Verification items for the finished model (mm, model axes). Face numbers are marked on the shaded views. A direction names the side the tool comes from. Give positions to 0.01 mm unless a question says otherwise; leave off trailing zeros. Order: outer loops, then holes, each group sorted by start corner. A loop starts at its lowest first (then second) coordinate and runs counter-clockwise, first axis right, second up. Notation, with made-up numbers: (2.25, 29) - (15.25, 29) arc R28 cw to (15.25, 47) - close; hole circle Ø11 at (12.5, -18). An arc over 180 degrees is marked (long way). Answer as a JSON object with one key per item and string values.
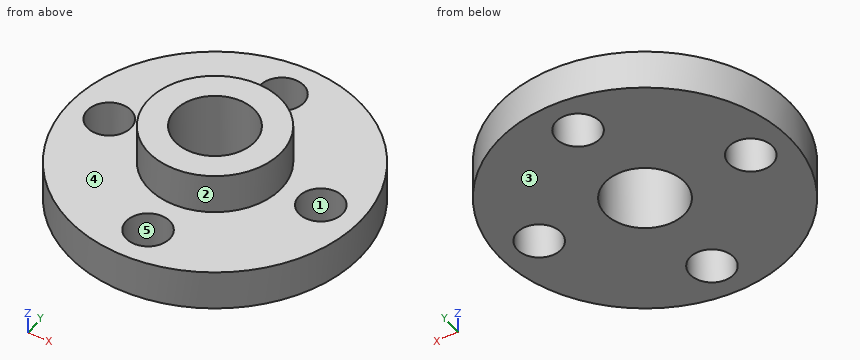
Autodesk Inventor part; units mm, degrees
ref_plane "YZ Plane" through (0, 0, 0) normal (1, 0, 0) x (0, 1, 0)
ref_plane "XZ Plane" through (0, 0, 0) normal (0, 1, 0) x (-1, 0, 0)
ref_plane "XY Plane" through (0, 0, 0) normal (0, 0, 1) x (1, 0, 0)
sketch "Sketch1" plane through (0, 0, 0) normal (0, 0, 1) x (1, 0, 0)
  circle A0 centre (0, 0) radius 11
  circle A1 centre (0, 8) radius 1.65
  line L0 (-3.4226, 0) -> (4.8397, 0) construction
  line L1 (0, 0) -> (0, 2.4255) construction
  circle A2 centre (8, 0) radius 1.65
  circle A3 centre (0, -8) radius 1.65
  circle A4 centre (-8, 0) radius 1.65
  dimension "d0" = 22
  dimension "d1" = 8
  dimension "d2" = 3.3
  dimension "d3" = 8
  dimension "d4" = 3.3
extrude "Extrusion1" add sketch "Sketch1" along normal blind 3
sketch "Sketch2" plane through (0, 0, 3) normal (0, 0, 1) x (1, 0, 0)
  circle A0 centre (0, 0) radius 5
  dimension "d7" = 10
extrude "Extrusion2" add sketch "Sketch2" along normal blind 3
sketch "Sketch3" plane through (0, 0, 6) normal (0, 0, 1) x (1, 0, 0)
  circle A0 centre (0, 0) radius 3
  dimension "d10" = 6
extrude "Extrusion3" cut sketch "Sketch3" against normal through all
equation "\"d4\" = d2"
properties part number "Acople" material "ABS Plastic"
(1) Section check D-D (y = 9). Record the cut outline in (x, z), then the cut area to 3 significant figures.
Computed values:
{"outline": "(-6.32, 0) - (-1.31, 0) - (-1.31, 3) - (-6.32, 3) - close; (1.31, 0) - (6.32, 0) - (6.32, 3) - (1.31, 3) - close", "area": "30.1 mm²"}
(2) Section check B-B (z = 0.65). Record the cut outline in (x, y), then the cut area to 3 significant figures.
Computed values:
{"outline": "circle Ø22 at (0, 0); hole circle Ø3.3 at (-8, 0); hole circle Ø6 at (0, 0); hole circle Ø3.3 at (0, -8); hole circle Ø3.3 at (0, 8); hole circle Ø3.3 at (8, 0)", "area": "318 mm²"}
(3) Gauge pin test, flat ends, axial feed: pin 1 Ø4.5 at (x, y) = (0, 8) entering from -Z; pin 2 Ø2 at (y, z) = (8, 3) entering from -X; pin 3 Ø4.5 at (x, y) = (0, -8) entering from +Z; pin 4 Ø1.5 at (y, z) = (7, 3) entering from -X. Record the tip position at first contact, or that the pin passes through.
Computed values:
{"pin 1": "stops at z = 0", "pin 2": "stops at x = -8.49", "pin 3": "stops at z = 3", "pin 4": "stops at x = -9.05"}
(4) Section check C-C (x = 8.25). Record the cut outline in (y, z).
Computed values:
{"outline": "(-7.28, 0) - (-1.63, 0) - (-1.63, 3) - (-7.28, 3) - close; (1.63, 0) - (7.28, 0) - (7.28, 3) - (1.63, 3) - close"}
(5) Section check A-A (x = 0). Record the cut outline in (y, z), then the cut area to 3 significant figures.
Computed values:
{"outline": "(-11, 0) - (-9.65, 0) - (-9.65, 3) - (-11, 3) - close; (-6.35, 0) - (-3, 0) - (-3, 6) - (-5, 6) - (-5, 3) - (-6.35, 3) - close; (3, 0) - (6.35, 0) - (6.35, 3) - (5, 3) - (5, 6) - (3, 6) - close; (9.65, 0) - (11, 0) - (11, 3) - (9.65, 3) - close", "area": "40.2 mm²"}
(6) Release check for a two-part mould opening along X. For the marked faces 1, 2 and 3 record: pulls with the +X half, pulls with the -X half, needs draft (parallel to the pull), parting line crosses it, or undercut.
Computed values:
{"face 1": "undercut", "face 2": "parting line crosses it", "face 3": "needs draft"}
(7) Material ranges on line 1 along Y through (x, z) = (0, 1.3); line 2 along X through (y, z) = (-1.25, 1.2); line 3 along X through (y, z) = (0.25, 2.4), recorded low to high. Write a range as [from, to].
Computed values:
{"line 1": "y = [-11, -9.65], [-6.35, -3], [3, 6.35], [9.65, 11]", "line 2": "x = [-10.93, -9.08], [-6.92, -2.73], [2.73, 6.92], [9.08, 10.93]", "line 3": "x = [-11, -9.63], [-6.37, -2.99], [2.99, 6.37], [9.63, 11]"}
(8) Access from +Z, -Z, +X, -X, +Y, -Y to the whole of each face (thin tool, end or side, straight path). Record for the marked faces 4 and 5.
Computed values:
{"face 4": "+Z", "face 5": "+Z, -Z"}
